from build123d import *

# Parameters (mm, degrees)
F3_DEPTH = 38.1
F4_R     = 3.175
F5_DEPTH = 76.2
F6_R     = 3.175
F7_DEPTH = 76.2
F8_R     = 3.175
F9_DEPTH = 76.2


with BuildPart() as f1:
    # F0 (on Front) → F1 (revolve)
    with BuildSketch(Plane.XZ):
        Polygon((101.6, 0), (25.4, 0), (25.4, -47.625), (31.75, -47.625), (31.75, -9.525), (101.6, -9.525), align=None)
    revolve(axis=Axis((0, 0, -4.0980735794), (0, 0, -1)))

    # F2 (on face) → F3 (join)
    with BuildSketch(Plane(origin=(0, 0, -9.525), x_dir=(1, 0, 0), z_dir=(0, 0, -1))):
        with BuildLine():
            Line((-28.575, 13.8395041457), (-28.575, 16.4977839421))
            Line((-28.575, 16.4977839421), (-98.7239970333, -24.0027583784))
            ThreePointArc((-98.7239970333, -24.0027583784), (-97.4517043144, -28.7354367675), (-95.952675689, -33.4012578824))
            Line((-95.952675689, -33.4012578824), (-31.5220452561, 3.7977839421))
            ThreePointArc((-31.5220452561, 3.7977839421), (-30.4651070619, 8.9409032938), (-28.575, 13.8395041457))
        make_face()
        with BuildLine():
            Line((-12.4720452561, -29.1977839421), (-76.902675689, -66.3968257666))
            ThreePointArc((-76.902675689, -66.3968257666), (-73.6114703867, -70.0279331946), (-70.1489970333, -73.4961102047))
            Line((-70.1489970333, -73.4961102047), (0, -32.9955678842))
            Line((0, -32.9955678842), (-2.302137834, -31.666427986))
            ThreePointArc((-2.302137834, -31.666427986), (-7.4895041457, -30.8540082915), (-12.4720452561, -29.1977839421))
        make_face()
        with BuildLine():
            ThreePointArc((2.302137834, -31.666427986), (0, -31.75), (-2.302137834, -31.666427986))
            Line((-2.302137834, -31.666427986), (0, -32.9955678842))
            Line((0, -32.9955678842), (2.302137834, -31.666427986))
        make_face()
        with BuildLine():
            ThreePointArc((70.1489970333, -73.4961102047), (73.6114703867, -70.0279331946), (76.902675689, -66.3968257666))
            Line((76.902675689, -66.3968257666), (12.4720452561, -29.1977839421))
            ThreePointArc((12.4720452561, -29.1977839421), (7.4895041457, -30.8540082915), (2.302137834, -31.666427986))
            Line((2.302137834, -31.666427986), (0, -32.9955678842))
            Line((0, -32.9955678842), (70.1489970333, -73.4961102047))
        make_face()
        with BuildLine():
            Line((98.7239970333, -24.0027583784), (28.575, 16.4977839421))
            Line((28.575, 16.4977839421), (28.575, 13.8395041457))
            ThreePointArc((28.575, 13.8395041457), (30.4651070619, 8.9409032938), (31.5220452561, 3.7977839421))
            Line((31.5220452561, 3.7977839421), (95.952675689, -33.4012578824))
            ThreePointArc((95.952675689, -33.4012578824), (97.4517043144, -28.7354367675), (98.7239970333, -24.0027583784))
        make_face()
        with BuildLine():
            ThreePointArc((-28.575, 13.8395041457), (-27.4963065702, 15.875), (-26.272862166, 17.8269238403))
            Line((-26.272862166, 17.8269238403), (-28.575, 16.4977839421))
            Line((-28.575, 16.4977839421), (-28.575, 13.8395041457))
        make_face()
        with BuildLine():
            Line((-19.05, 25.4), (-19.05, 99.7980836489))
            ThreePointArc((-19.05, 99.7980836489), (-23.8402339277, 98.7633699621), (-28.575, 97.4988685832))
            Line((-28.575, 97.4988685832), (-28.575, 16.4977839421))
            Line((-28.575, 16.4977839421), (-26.272862166, 17.8269238403))
            ThreePointArc((-26.272862166, 17.8269238403), (-22.9756029161, 21.9131049977), (-19.05, 25.4))
        make_face()
        with BuildLine():
            Line((28.575, 16.4977839421), (26.272862166, 17.8269238403))
            ThreePointArc((26.272862166, 17.8269238403), (27.4963065702, 15.875), (28.575, 13.8395041457))
            Line((28.575, 13.8395041457), (28.575, 16.4977839421))
        make_face()
        with BuildLine():
            ThreePointArc((28.575, 97.4988685832), (23.8402339277, 98.7633699621), (19.05, 99.7980836489))
            Line((19.05, 99.7980836489), (19.05, 25.4))
            ThreePointArc((19.05, 25.4), (22.9756029161, 21.9131049977), (26.272862166, 17.8269238403))
            Line((26.272862166, 17.8269238403), (28.575, 16.4977839421))
            Line((28.575, 16.4977839421), (28.575, 97.4988685832))
        make_face()
    extrude(amount=F3_DEPTH)

    # F4 (on face) → F5 (cut)
    with BuildSketch(Plane.YZ.offset(28.575)):
        with Locations((-87.9738685832, -34.925)):
            Circle(F4_R)
    extrude(amount=-F5_DEPTH, mode=Mode.SUBTRACT)

    # F6 (on face) → F7 (cut)
    with BuildSketch(Plane(origin=(14.2875, -24.7466759131, 0), x_dir=(0.8660254038, 0.5, 0), z_dir=(0.5, -0.8660254038, 0))):
        with Locations((84.7988685832, -34.925)):
            Circle(F6_R)
    extrude(amount=-F7_DEPTH, mode=Mode.SUBTRACT)

    # F8 (on face) → F9 (cut)
    with BuildSketch(Plane(origin=(-14.2875, -24.7466759131, 0), x_dir=(0.8660254038, -0.5, 0), z_dir=(-0.5, -0.8660254038, 0))):
        with Locations((-84.7988685832, -34.925)):
            Circle(F8_R)
    extrude(amount=-F9_DEPTH, mode=Mode.SUBTRACT)


solid = f1.part
Part model, mm, in its own coordinate system. A direction names the side the tool comes from. Round coordinates to 2 decimals unless told otherwise and drop trailing zeros. Write each loop counter-clockwise with the first axis right and the second up, starting at its lowest first coordinate (ties: lowest second). Pieces come first, ordered by that corner, then holes. Notation, with made-up numbers: M 18.5,-27.75 L 54.5,-27.75 A18 ccw 54.5,-0.75 Z; hole C 81,-1.5 d3. An arc over 180 degrees is marked long. Return JSON: item names as keys, results as strings. Group by question number.
(1) Pin check, flat tips, straight feed: pin 1 Ø2 at (y, z) = (-18, -19) entering from -X (3 decimals); pin 2 Ø10 at (y, z) = (-87.97, -34.92) entering from +X (3 decimals); pin 3 Ø19 at (x, y) = (-7.5, -80.5) entering from -Z (3 decimals); pin 4 Ø4 at (y, z) = (-87.97, -34.92) entering from +X. Stop position of each tip, or through.
(2) Which spindle directions (+Z, -Z, +X, -X, +Y, -Y) get a long thin tool onto all of the face, cutting with end or side? Do faces 4 (the face through (-64.188, 15.062, -28.308)), 5 (the face through (19.05, -63, -28)), 6 (the face through (-59.025, 61.497, -36.141)). Say none if no direction does.
(3) Saw through at A-A on z = -13. Write the cut outline in (x, y) (3 decimals), then the cut area to 3 significant figures.
(4) Two-plate mould, pull along Y, no slides. Class faces 1 (the face through (34.58, 52.96, -28.31)), 2 (the face through (64.105, 64.43, -36.141)), 3 (the face through (66, -38, -9.525)): +Y half, -Y half, draft (parallel to the pull), parting line (faces both ways), or undercut.
(5) Saw through at B-B on x = -5.5. Write the cut outline in (y, z) (3 decimals).
(6) Saw through at C-C on y = 0. Write the cut outline in (x, z) (3 decimals), then the cut area to 3 significant figures.
(7) Saw through at D-D on x = 40.5. Write the cut outline in (y, z) (3 decimals).
(8) Drill centre lines: probe 1 along X at (y, z) = (-76, -31.5) (3 decimals); probe 2 along Y at (x, z) = (19, -15); probe 3 along Y at (x, z) = (16, -35). Where is each one in solid material? Low to high.
Returned:
{
 "1": {"pin 1": "x = -28.575", "pin 2": "x = 28.575", "pin 3": "z = -9.525", "pin 4": "through"},
 "2": {"face 4": "-Z", "face 5": "-Z, -Y", "face 6": "none"},
 "3": {"outline": "M -98.724,24.003 L -28.575,-16.498 L -28.575,-97.499 A101.6 ccw -19.05,-99.798 L -19.05,-25.4 A31.75 ccw 19.05,-25.4 L 19.05,-99.798 A101.6 ccw 28.575,-97.499 L 28.575,-16.498 L 98.724,24.003 A101.6 ccw 95.953,33.401 L 31.522,-3.798 A31.75 ccw 12.472,29.198 L 76.903,66.397 A101.6 ccw 70.149,73.496 L 0,32.996 L -70.149,73.496 A101.6 ccw -76.903,66.397 L -12.472,29.198 A31.75 ccw -31.522,-3.798 L -95.953,33.401 A101.6 ccw Z; hole C 0,0 d50.8", "area": "5,600 mm²"},
 "4": {"face 1": "+Y half", "face 2": "undercut", "face 3": "draft"},
 "5": {"outline": "M -101.451,-9.525 L -31.27,-9.525 L -31.27,-47.625 L -24.797,-47.625 L -24.797,0 L -101.451,0 Z; M 24.797,-47.625 L 36.171,-47.625 L 36.171,-9.525 L 101.451,-9.525 L 101.451,0 L 24.797,0 Z"},
 "6": {"outline": "M -101.6,-9.525 L -57.15,-9.525 L -57.15,-47.625 L -38.1,-47.625 L -38.1,-9.525 L -31.75,-9.525 L -31.75,-47.625 L -25.4,-47.625 L -25.4,0 L -101.6,0 Z; M 25.4,-47.625 L 31.75,-47.625 L 31.75,-9.525 L 38.1,-9.525 L 38.1,-47.625 L 57.15,-47.625 L 57.15,-9.525 L 101.6,-9.525 L 101.6,0 L 25.4,0 Z", "area": "3,390 mm²"},
 "7": {"outline": "M -93.179,-9.525 L -9.613,-9.525 L -9.613,-47.625 L 1.386,-47.625 L 1.386,-9.525 L 45.38,-9.525 L 45.38,-47.625 L 56.378,-47.625 L 56.378,-9.525 L 93.179,-9.525 L 93.179,0 L -93.179,0 Z"},
 "8": {"probe 1": "-28.575 to -19.05, 19.05 to 28.575", "probe 2": "-25.44 to -16.86, 16.86 to 25.44, 32.97 to 43.97", "probe 3": "-27.42 to -19.73, 19.73 to 27.42, 31.23 to 42.23"}
}
